```python
from build123d import *

# Parameters (mm, degrees)
BOSS_EXTRUDE1_DEPTH = 15.24
BOSS_EXTRUDE2_DEPTH = 2.54
BOSS_EXTRUDE3_DEPTH = 15.24
CUT_EXTRUDE3_DEPTH  = 15.24
FILLET9_R           = 2.54
CUT_EXTRUDE4_DEPTH  = 15.24
FILLET1_R           = 2.54


with BuildPart() as part:
    # Sketch1 → Boss-Extrude1 (new body)
    with BuildSketch(Plane(origin=(0, 0, 0), x_dir=(1, 0, 0), z_dir=(0, 1, 0))):
        Polygon((10.705228691, 0), (5.352614346, 9.271), (-5.352614346, 9.271), (-10.705228691, 0), (-5.352614346, -9.271), (5.352614346, -9.271), align=None)
        Polygon((7.772289324, 0), (3.886144662, 6.731), (-3.886144662, 6.731), (-7.772289324, 0), (-3.886144662, -6.731), (3.886144662, -6.731), align=None, mode=Mode.SUBTRACT)
    extrude(amount=BOSS_EXTRUDE1_DEPTH)

    # Sketch2 → Boss-Extrude2 (add)
    with BuildSketch(Plane(origin=(0, 15.24, 0), x_dir=(1, 0, 0), z_dir=(0, 1, 0))):
        Polygon((10.705228691, 0), (5.352614346, 9.271), (-5.352614346, 9.271), (-10.705228691, 0), (-5.352614346, -9.271), (5.352614346, -9.271), align=None)
    extrude(amount=BOSS_EXTRUDE2_DEPTH)

    # Sketch3 → Boss-Extrude3 (add)
    with BuildSketch(Plane(origin=(0, 17.78, 0), x_dir=(1, 0, 0), z_dir=(0, 1, 0))):
        Polygon((4.399409051, 0), (2.199704526, 3.81), (-2.199704526, 3.81), (-4.399409051, 0), (-2.199704526, -3.81), (2.199704526, -3.81), align=None)
    extrude(amount=BOSS_EXTRUDE3_DEPTH)

    # Sketch8 → Cut-Extrude3 (cut)
    with BuildSketch(Plane.XZ):
        with BuildLine():
            Line((3.886144662, 6.731), (7.772289324, 0))
            add(Edge.make_bspline(
                [(3.886144662, 6.731), (7.588980613, 4.3815), (7.772289324, 0)],
                knots=[0, 0, 0, 1, 1, 1], degree=2))
        make_face()
    extrude(amount=-CUT_EXTRUDE3_DEPTH, mode=Mode.SUBTRACT)

    # Fillet9
    fillet9_edges = [part.edges().sort_by_distance(p)[0] for p in [
        (3.299556788, 17.78, 1.905),
        (3.299556788, 17.78, -1.905),
        (0, 17.78, -3.81),
        (-3.299556788, 17.78, -1.905),
        (-3.299556788, 17.78, 1.905),
        (0, 17.78, 3.81),
        (3.299556788, 33.02, 1.905),
        (3.299556788, 33.02, -1.905),
        (0, 33.02, -3.81),
        (-3.299556788, 33.02, -1.905),
        (-3.299556788, 33.02, 1.905),
        (0, 33.02, 3.81),
    ]]
    fillet(fillet9_edges, radius=FILLET9_R)

    # Sketch9 → Cut-Extrude4 (cut)
    with BuildSketch(Plane.XZ):
        with BuildLine():
            Line((-7.772289324, 0), (-3.886144662, -6.731))
            add(Edge.make_bspline(
                [(-7.772289324, 0), (-7.588980613, -4.3815), (-3.886144662, -6.731)],
                knots=[0, 0, 0, 1, 1, 1], degree=2))
        make_face()
    extrude(amount=-CUT_EXTRUDE4_DEPTH, mode=Mode.SUBTRACT)

    # Fillet1
    fillet1_edges = [part.edges().sort_by_distance(p)[0] for p in [
        (8.028921518, 17.78, 4.6355),
        (8.028921518, 17.78, -4.6355),
        (0, 17.78, -9.271),
        (-8.028921518, 17.78, -4.6355),
        (-8.028921518, 17.78, 4.6355),
        (0, 17.78, 9.271),
    ]]
    fillet(fillet1_edges, radius=FILLET1_R)


solid = part.part
```
The model under review builds one solid part; all positions refer to its coordinate system, in mm. A direction names the side the tool comes from. Round coordinates to 2 decimals unless told otherwise and drop trailing zeros. Loops run counter-clockwise (first coordinate to the right, second up) from the corner with the lowest first, then second, coordinate; pieces in that order, holes last.
1) Tool access review of faces 1 (the face through (3.315, 25.329, -1.878)), 2 (the face through (-7.99, 7.51, -4.7)), 3 (the face through (3.284, 25.329, 1.932)): name each direction out of +Z, -Z, +X, -X, +Y, -Y from which nothing blocks a thin tool from reaching the whole face with its end or side.
Values follow:
face 1: -Z, +X, +Y
face 2: -Z, -X, +Y, -Y
face 3: +Z, +X, +Y
2) Clearance check with flat-ended pins moving along their axes: P1, Ø1, axis at y = 13, z = -6.5, coming from the +X side; P2, Ø1, axis at y = 25.5, z = 3, coming from the +X side; P3, Ø4, axis at x = -4.5, y = 21.5, coming from the -Z side. State where each tip first meets the part, or that it passes through.
Values follow:
P1: stops at x = 7.24
P2: stops at x = 2.96
P3: stops at z = -3.29
3) Wall thickness on line 1 along Z through (x, y) = (-3.5, 1.5); line 2 along Y through (x, z) = (1, -0.5); line 3 along Y through (x, z) = (6.25, -2.5): over which ranges is each line inside the solid? List them lowest first.
Values follow:
line 1: z = -9.27 to -6.73, 6.73 to 9.27
line 2: y = 15.24 to 33.02
line 3: y = 15.24 to 17.78
4) Consider section A-A on y = 25. State the section outline as (x, z) points.
Values follow:
outline: (-4.4, 0) - (-2.2, -3.81) - (2.2, -3.81) - (4.4, 0) - (2.2, 3.81) - (-2.2, 3.81) - close
